Geometry check sheet. Reference: the model listing, model coordinates, mm. A direction names the side the tool comes from. Give positions to 0.01 mm unless a question says otherwise; leave off trailing zeros. Order: outer loops, then holes, each group sorted by start corner. A loop starts at its lowest first (then second) coordinate and runs counter-clockwise, first axis right, second up.
Autodesk Fusion 360 part; units mm, degrees
sketch "Sketch1" plane through (0, 0, 0) normal (0, 1, 0) x (1, 0, 0)
  line L0 (0, 0) -> (30, 0)
  line L1 (30, 0) -> (30, -11.5)
  line L2 (30, -11.5) -> (0, -11.5)
  line L3 (0, -11.5) -> (0, 0)
  dimension "d1" = 30
  dimension "d2" = 11.5
extrude "Extrude1" add sketch "Sketch1" along normal blind 4.5

Autodesk Fusion 360 part; units mm, degrees
sketch "Sketch1" plane through (0, 0, 0) normal (0, 1, 0) x (1, 0, 0)
  line L0 (0, 0) -> (17.5, 0)
  line L1 (17.5, 0) -> (17.5, 3)
  line L2 (17.5, 3) -> (0, 3)
  line L3 (0, 3) -> (0, 0)
  line L4 (0, 0) -> (1, 0)
  line L5 (17.5, 0) -> (16.5, 0)
  line L6 (0, 3) -> (8.75, 3)
  line L7 (0, 0) -> (0, 1)
  line L8 (17.5, 0) -> (17.5, 1)
  line L9 (8.75, 3) -> (8.75, 2)
  spline S0 degree 5 poles (0, 1) (-0.0052, 0.8576) (0.0051, 0.5979) (0.0824, 0.284) (0.3098, 0.0171) (0.8015, -0.0688) (1.4966, 0.0725) (2.3822, 0.3921) (3.4374, 0.8195) (4.6351, 1.2741) (5.9435, 1.6748) (7.3276, 1.9503) (8.75, 2.049) (10.1724, 1.9503) (11.5565, 1.6748) (12.8649, 1.2741) (14.0626, 0.8195) (15.1178, 0.3921) (16.0034, 0.0725) (16.6985, -0.0688) (17.1902, 0.0171) (17.4176, 0.284) (17.4949, 0.5979) (17.5052, 0.8576) (17.5, 1) knots 0 0 0 0 0 0 0.05 0.1 0.15 0.2 0.25 0.3 0.35 0.4 0.45 0.5 0.55 0.6 0.65 0.7 0.75 0.8 0.85 0.9 0.95 1 1 1 1 1 1
  line L10 (17.5, 3) -> (0, 3)
  line L11 (0, 3) -> (0, 4.5)
  line L12 (0, 4.5) -> (17.5, 4.5)
  line L13 (17.5, 4.5) -> (17.5, 3)
  dimension "d1" = 17.5
  dimension "d2" = 3
  dimension "d3" = 1
  dimension "d4" = 1
  dimension "d5" = 8.75
  dimension "d6" = 1
  dimension "d7" = 1
  dimension "d8" = 1
  dimension "d23" = 17.5
  dimension "d24" = 1.5
extrude "Extrude1" add sketch "Sketch1" along normal blind 4 contours L0 L3 L4 L7 S0 | L0 L2 L3 L4 L6 L9 S0 L10 | L0 L1 L5 L8 S0 | L0 L1 L2 L5 L9 S0 L10 | L2 L6 L10 L11 L12 L13
draft "Draft1" angle 7.5 neutral plane through (0, 4, 0) pull (0, 1, 0) 1 faces at (5.8333, 2.6667, -4.5)
sketch "Sketch3" plane through (0, 0.6505, -4.941) normal (0, 0.1305, -0.9914) x (-1, 0, 0)
  line L0 (-17.5, -0.6561) -> (0, -0.6561)
  line L1 (0, -0.6561) -> (0, 3.3784)
  line L2 (0, 3.3784) -> (-17.5, 3.3784)
  line L3 (-17.5, 3.3784) -> (-17.5, -0.6561)
  line L4 (-17.5, 3.3784) -> (-16.25, 3.3784)
  line L5 (-16.25, 3.3784) -> (-16.25, 2.1284)
  line L6 (-16.25, 2.1284) -> (-17.5, 2.1284)
  line L7 (-17.5, 2.1284) -> (-17.5, 3.3784)
  line L8 (-16.25, 2.1284) -> (-1.25, 2.1284)
  line L9 (-1.25, 2.1284) -> (-1.25, -0.6561)
  line L10 (-1.25, -0.6561) -> (-16.25, -0.6561)
  line L11 (-16.25, -0.6561) -> (-16.25, 2.1284)
  line L12 (-1.25, 2.1284) -> (0, 2.1284)
  line L13 (-1.25, 2.1284) -> (-1.25, 3.3784)
  line L14 (-16.25, 3.3784) -> (-1.25, 3.3784)
  line L15 (-1.25, 3.3784) -> (-1.25, 4.3784)
  line L16 (-1.25, 4.3784) -> (-16.25, 4.3784)
  line L17 (-16.25, 4.3784) -> (-16.25, 3.3784)
  dimension "d25" = 1.25
  dimension "d26" = 1.25
  dimension "d34" = 1
extrude "Extrude3" cut sketch "Sketch3" against normal blind 1.5 contours L0 L8 L9 L10 L11
extrude "Extrude4" cut sketch "Sketch3" against normal blind 0.5 contours L2 L5 L8 L13 L14 | L2 L14 L15 L16 L17
fillet "Fillet1" [suppressed]
Item 1: Gauge pin test, flat end, axial feed: pin 1 (1.5 mm diameter, centred on x = 5.5, y = 2.5, fed in from -Z). Record the tip position at first contact, or that the pin passes through.
Reported:
pin 1: stops at z = -4.17
Item 2: Sectioned sample at A-A (x = 2.5). Enter the section's corners in (y, z).
Reported:
outline: (0, -3.51) - (2.56, -3.18) - (2.7, -4.17) - (4.5, -3.93) - (4.5, 0) - (0, 0) - close
Item 3: Set-up check for faces 1 (the flat face through (9, 2, 0)), 2 (the flat face through (8.855, 3.61, -4.047)), 3 (the flat face through (8.855, 1.3, -3.342)), 4 (the flat face through (0, 2, -3)), 5 (the flat face through (9, 4.5, -2)): record each of +Z, -Z, +X, -X, +Y, -Y from which the full face is reachable in a straight line by a thin tool's end or side.
Reported:
face 1: +Z, +Y, -Y
face 2: -Z, +Y
face 3: -Z
face 4: +Z, -Z, -X, +Y, -Y
face 5: +Z, -Z, +X, -X, +Y
Item 4: Scan lines: L1, parallel to X at y = 3.5, z = -4.3; L2, parallel to Z at x = 12.5, y = 1.3; L3, parallel to Z at x = 9.75, y = 0.75. Record each from-to range of solid material in increasing order.
Reported:
L1: x = 0 to 1.25, 16.25 to 17.5
L2: z = -3.34 to 0
L3: z = -3.41 to 0
Item 5: Draft check along X on faces 6 (the flat face through (9, 0, -2)), 7 (the flat face through (16.25, 2, -4)), 8 (the flat face through (17.5, 2, -2)). Enter one of: released by +X, released by -X, zero draft, split by the parting line, or undercut.
Reported:
face 6: zero draft
face 7: undercut
face 8: released by +X
